Part model, mm, in its own coordinate system. Round coordinates to 2 decimals unless told otherwise and drop trailing zeros. Write each loop counter-clockwise with the first axis right and the second up, starting at its lowest first coordinate (ties: lowest second). Pieces come first, ordered by that corner, then holes. Notation, with made-up numbers: M 37.25,8 L 73.25,8 A26 ccw 73.25,22 Z; hole C 46.25,70.5 d11. An arc over 180 degrees is marked long. Answer as a JSON object with one key per item and string values. Group by question number.
1. Drop flat-ended pins along their axis: pin 1 (0.7 mm diameter, centred on y = 35.5, z = 1.5, fed in from +X); pin 2 (20 mm diameter, centred on x = 28.5, y = -19.5, fed in from +Z); pin 3 (1.1 mm diameter, centred on y = 57, z = 1, fed in from +X); pin 4 (1.7 mm diameter, centred on x = 3, y = -57, fed in from -Z). Give the stop position or say it passes through.
2. Two-plate mould, pull along Y, no slides. Class faces 1 (the face through (25, -19, 1)), 2 (the face through (94, 1, 2.2)): +Y half, -Y half, draft (parallel to the pull), parting line (faces both ways), or undercut.
3. Drill centre lines: line 1 (Y direction, x = 27, z = 1.5); line 2 (X direction, y = -36.5, z = 1.95); line 3 (Y direction, x = 44, z = 1.9). Where is each one in solid material? Low to high. Write a range as from..to.
4. Band-saw the part on C-C, the plane y = -28. Write the cut outline in (x, z).
5. Band-saw the part on B-B, the plane z = 0.5. Count the separate pieces of the cut face and the enclosed holes in it, plus the area to 3 significant figures.
6. Band-saw the part on A-A, the plane x = 18. Write the cut outline in (y, z), plus the area to 3 significant figures.
7. Band-saw the part on D-D, the plane x = 108. Write the cut outline in (y, z), plus the area to 3 significant figures.
from build123d import *

# Parameters (mm, degrees)
BOSS_EXTRUDE1_DEPTH                            = 2.2
CSK_FOR_M2_5_COUNTERSUNK_FLAT_HEAD_S_2_COUNT   = 2
CSK_FOR_M2_5_COUNTERSUNK_FLAT_HEAD_S_2_PITCH   = 76.225
CSK_FOR_M2_5_COUNTERSUNK_FLAT_HEAD_S_3_COUNT   = 2
CSK_FOR_M2_5_COUNTERSUNK_FLAT_HEAD_S_3_PITCH   = 85.216551356
CSK_FOR_M2_5_COUNTERSUNK_FLAT_HEAD_S_4_COUNT   = 2
CSK_FOR_M2_5_COUNTERSUNK_FLAT_HEAD_S_4_PITCH   = 38.1
CSK_FOR_M2_5_COUNTERSUNK_FLAT_HEAD_S_5_A_COUNT = 2
CSK_FOR_M2_5_COUNTERSUNK_FLAT_HEAD_S_5_A_PITCH = 24
CSK_FOR_M2_5_COUNTERSUNK_FLAT_HEAD_S_6_COUNT   = 2
CSK_FOR_M2_5_COUNTERSUNK_FLAT_HEAD_S_6_PITCH   = 114
CSK_FOR_M2_5_COUNTERSUNK_FLAT_HEAD_S_7_COUNT   = 2
CSK_FOR_M2_5_COUNTERSUNK_FLAT_HEAD_S_7_PITCH   = 116.498927034
CUT_EXTRUDE1_DEPTH                             = 167.222260844
CUT_EXTRUDE1_DEPTH_BACK                        = 1.2
SKETCH4_W                                      = 40
SKETCH4_H                                      = 69


with BuildPart() as part:
    # Sketch1 → Boss-Extrude1 (new body)
    with BuildSketch(Plane.XY):
        with BuildLine():
            Line((2, -60), (28, -60))
            ThreePointArc((28, -60), (29.414213562, -59.414213562), (30, -58))
            Line((30, -58), (30, -55))
            Line((30, -55), (153, -55))
            ThreePointArc((153, -55), (154.414213562, -54.414213562), (155, -53))
            Line((155, -53), (155, 17.5))
            Line((155, 17.5), (149.5, 17.5))
            Line((149.5, 17.5), (149.5, 55))
            Line((149.5, 55), (30, 55))
            Line((30, 55), (30, 58))
            ThreePointArc((30, 58), (29.414213562, 59.414213562), (28, 60))
            Line((28, 60), (2, 60))
            ThreePointArc((2, 60), (0.585786438, 59.414213562), (0, 58))
            Line((0, 58), (0, -58))
            ThreePointArc((0, -58), (0.585786438, -59.414213562), (2, -60))
        make_face()
    extrude(amount=BOSS_EXTRUDE1_DEPTH)

    # Sketch2 → CSK for M2.5 Countersunk Flat Head Screw (revolve, cut)
    with BuildSketch(Plane(origin=(52.575, 28.25, 0), x_dir=(0, 1, 0), z_dir=(1, 0, 0))):
        Polygon((0, 0), (0, 2.2), (1.45, 2.2), (1.45, 1.3), (2.75, 0), align=None)
    csk_for_m2_5_countersunk_flat_head_screw = revolve(axis=Axis((52.575, 28.25, -6.35), (0, 0, 1)), mode=Mode.SUBTRACT)

    # CSK for M2.5 Countersunk Flat Head S 2: CSK for M2.5 Countersunk Flat Head Screw ×2
    with Locations(*[(i * CSK_FOR_M2_5_COUNTERSUNK_FLAT_HEAD_S_2_PITCH, 0, 0) for i in range(1, CSK_FOR_M2_5_COUNTERSUNK_FLAT_HEAD_S_2_COUNT)]):
        add(csk_for_m2_5_countersunk_flat_head_screw, mode=Mode.SUBTRACT)

    # CSK for M2.5 Countersunk Flat Head S 3: CSK for M2.5 Countersunk Flat Head Screw ×2
    with Locations(*[Vector(0.8944858573496409, -0.4470962435555436, 0) * (i * CSK_FOR_M2_5_COUNTERSUNK_FLAT_HEAD_S_3_PITCH) for i in range(1, CSK_FOR_M2_5_COUNTERSUNK_FLAT_HEAD_S_3_COUNT)]):
        add(csk_for_m2_5_countersunk_flat_head_screw, mode=Mode.SUBTRACT)

    # CSK for M2.5 Countersunk Flat Head S 4: CSK for M2.5 Countersunk Flat Head Screw ×2
    with Locations(*[(0, -i * CSK_FOR_M2_5_COUNTERSUNK_FLAT_HEAD_S_4_PITCH, 0) for i in range(1, CSK_FOR_M2_5_COUNTERSUNK_FLAT_HEAD_S_4_COUNT)]):
        add(csk_for_m2_5_countersunk_flat_head_screw, mode=Mode.SUBTRACT)

    # Sketch3 → CSK for M2.5 Countersunk Flat Head S 5 (revolve, cut)
    with BuildSketch(Plane(origin=(27, 57, 0), x_dir=(0, 1, 0), z_dir=(1, 0, 0))):
        Polygon((0, 0), (0, 2.2), (1.45, 2.2), (1.45, 1.3), (2.75, 0), align=None)
    csk_for_m2_5_countersunk_flat_head_s_5 = revolve(axis=Axis((27, 57, -6.35), (0, 0, 1)), mode=Mode.SUBTRACT)

    # CSK for M2.5 Countersunk Flat Head S 5 a: CSK for M2.5 Countersunk Flat Head S 5 ×2
    with Locations(*[(-i * CSK_FOR_M2_5_COUNTERSUNK_FLAT_HEAD_S_5_A_PITCH, 0, 0) for i in range(1, CSK_FOR_M2_5_COUNTERSUNK_FLAT_HEAD_S_5_A_COUNT)]):
        add(csk_for_m2_5_countersunk_flat_head_s_5, mode=Mode.SUBTRACT)

    # CSK for M2.5 Countersunk Flat Head S 6: CSK for M2.5 Countersunk Flat Head S 5 ×2
    with Locations(*[(0, -i * CSK_FOR_M2_5_COUNTERSUNK_FLAT_HEAD_S_6_PITCH, 0) for i in range(1, CSK_FOR_M2_5_COUNTERSUNK_FLAT_HEAD_S_6_COUNT)]):
        add(csk_for_m2_5_countersunk_flat_head_s_5, mode=Mode.SUBTRACT)

    # CSK for M2.5 Countersunk Flat Head S 7: CSK for M2.5 Countersunk Flat Head S 5 ×2
    with Locations(*[Vector(-0.206010481049842, -0.978549784986749, 0) * (i * CSK_FOR_M2_5_COUNTERSUNK_FLAT_HEAD_S_7_PITCH) for i in range(1, CSK_FOR_M2_5_COUNTERSUNK_FLAT_HEAD_S_7_COUNT)]):
        add(csk_for_m2_5_countersunk_flat_head_s_5, mode=Mode.SUBTRACT)

    # Sketch4 → Cut-Extrude1 (cut, two sides: drawn at the far end of the back side and taken through both)
    with BuildSketch(Plane.XY.offset(2.2).offset(-CUT_EXTRUDE1_DEPTH_BACK)):
        with Locations((25, -19)):
            Rectangle(SKETCH4_W, SKETCH4_H)
    extrude(amount=CUT_EXTRUDE1_DEPTH + CUT_EXTRUDE1_DEPTH_BACK, mode=Mode.SUBTRACT)


solid = part.part
Worked answers:
{
 "1": {"pin 1": "stops at x = 149.5", "pin 2": "stops at z = 1", "pin 3": "stops at x = 30", "pin 4": "passes through"},
 "2": {"face 1": "undercut", "face 2": "draft"},
 "3": {"line 1": "y = -60..-58.45, -55.55..-53.5, 15.5..55.55, 58.45..60", "line 2": "x = 0..5, 45..155", "line 3": "y = -55..-53.5, 15.5..55"},
 "4": {"outline": "M 0,0 L 155,0 L 155,2.2 L 45,2.2 L 45,1 L 5,1 L 5,2.2 L 0,2.2 Z"},
 "5": {"separate pieces": "1", "enclosed holes": "8", "area": "17,000 mm^2"},
 "6": {"outline": "M -60,0 L 60,0 L 60,2.2 L 15.5,2.2 L 15.5,1 L -53.5,1 L -53.5,2.2 L -60,2.2 Z", "area": "181 mm^2"},
 "7": {"outline": "M -55,0 L 55,0 L 55,2.2 L -55,2.2 Z", "area": "242 mm^2"}
}
